Input: dimensioned drawing with shaded views. Units: mm. Origin: part minimum x, y, z. A direction names the side the tool comes from. Round coordinates to 2 decimals unless told otherwise and drop trailing zeros. Loops run counter-clockwise (first coordinate to the right, second up) from the corner with the lowest first, then second, coordinate; pieces in that order, holes last. Notation, with made-up numbers: (79.5, -13.75) - (98.5, -13.75) arc R18 ccw to (98.5, 15.25) - close; hole circle Ø6 at (14.25, 82). An arc over 180 degrees is marked (long way). Write each question's results on one line, items separated by ' | '.
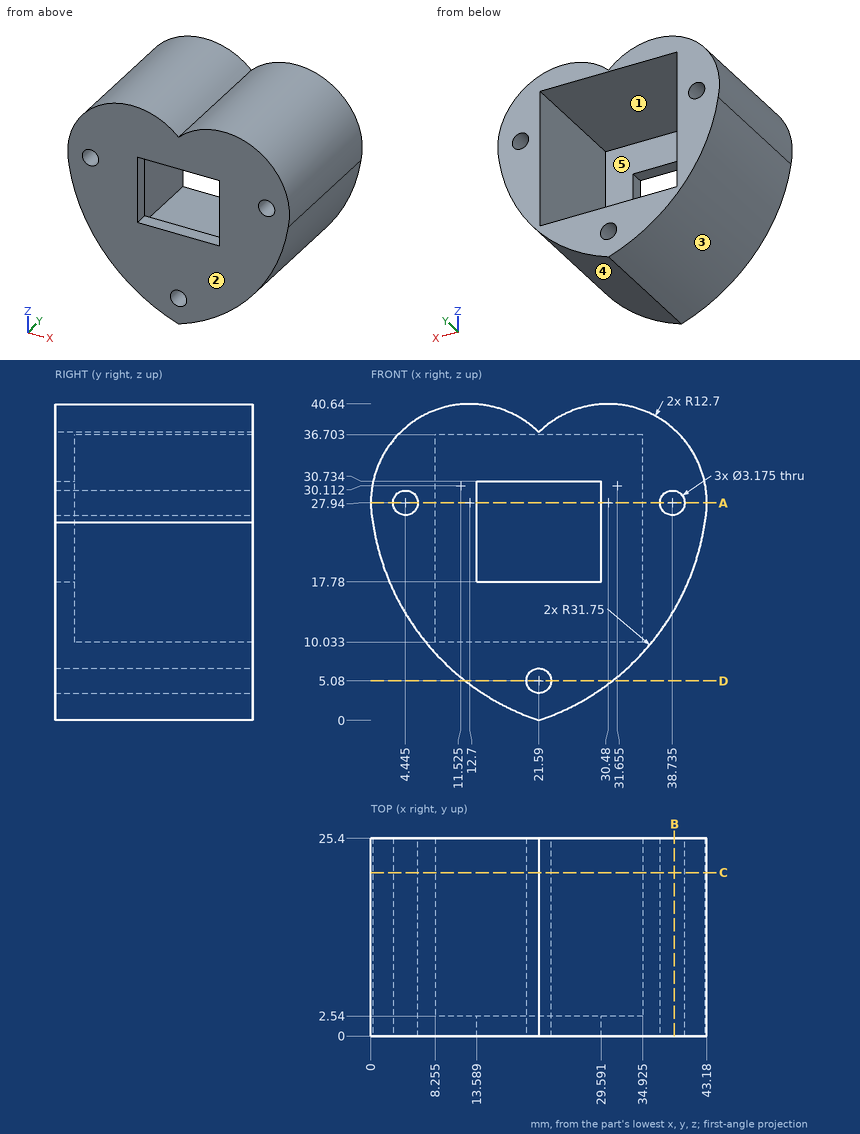
1. Mould query, pull axis Z, two halves, no side actions, for the marked faces 1, 2 and 3. Classes: pulls with the +Z half, pulls with the -Z half, needs draft (parallel to the pull), parting line crosses it, or undercut.
Answer:
face 1: undercut | face 2: needs draft | face 3: pulls with the -Z half
2. Section query C-C, the plane y = 21. Count the separate pieces of the cut face and the enclosed holes in it, plus the area to 3 significant figures.
Answer:
separate pieces: 1 | enclosed holes: 4 | area: 585 mm^2
3. Set-up query: the marked faces 4 and 5. Return all of +Z, -Z, +X, -X, +Y, -Y with unobstructed straight access to the full face (end or side cutting, diameter ignored); none if empty.
Answer:
face 4: -Z, +X, +Y, -Y | face 5: +Y
4. Contact query for flat-ended pins moving along their axis: pin 1 (2 mm diameter, centred on x = 19.5, y = 1, fed in from +Z); pin 2 (2 mm diameter, centred on x = 18.5, y = 9.5, fed in from +Z); pin 3 (2 mm diameter, centred on y = 2.5, z = 12.5, fed in from +X); pin 4 (2 mm diameter, centred on x = 21.5, y = 0.5, fed in from -Z). Output: stop coordinate, or through.
Answer:
pin 1: z = 39.24 | pin 2: z = 39.7 | pin 3: x = 38.58 | pin 4: z = 0
5. Section query B-B, the plane x = 39. Output: boundary loops of the cut face in (y, z) (1 decimal).
Answer:
outline: (0, 14.2) - (25.4, 14.2) - (25.4, 26.4) - (0, 26.4) - close; (0, 29.5) - (25.4, 29.5) - (25.4, 37.4) - (0, 37.4) - close
6. Section query A-A, the plane z = 27.94. Output: boundary loops of the cut face in (x, y) (1 decimal).
Answer:
outline: (0, 0) - (2.9, 0) - (2.9, 25.4) - (0, 25.4) - close; (6, 0) - (13.6, 0) - (13.6, 2.5) - (8.3, 2.5) - (8.3, 25.4) - (6, 25.4) - close; (29.6, 0) - (37.1, 0) - (37.1, 25.4) - (34.9, 25.4) - (34.9, 2.5) - (29.6, 2.5) - close; (40.3, 0) - (43.2, 0) - (43.2, 25.4) - (40.3, 25.4) - close
7. Line query: line 1 (X direction, y = 23.75, z = 28) (1 decimal); line 2 (Z direction, x = 20.5, y = 9) (1 decimal); line 3 (Y direction, x = 34.5, z = 21). Output: solid intervals per line, ascending. Write a range as [from, to].
Answer:
line 1: [0, 2.9], [6, 8.3], [34.9, 37.1], [40.3, 43.2] | line 2: [0.4, 3.9], [6.2, 10], [36.7, 38] | line 3: [0, 2.54]
8. Section query D-D, the plane z = 5.08. Output: boundary loops of the cut face in (x, y) (1 decimal).
Answer:
outline: (12.1, 0) - (20, 0) - (20, 25.4) - (12.1, 25.4) - close; (23.2, 0) - (31.1, 0) - (31.1, 25.4) - (23.2, 25.4) - close
